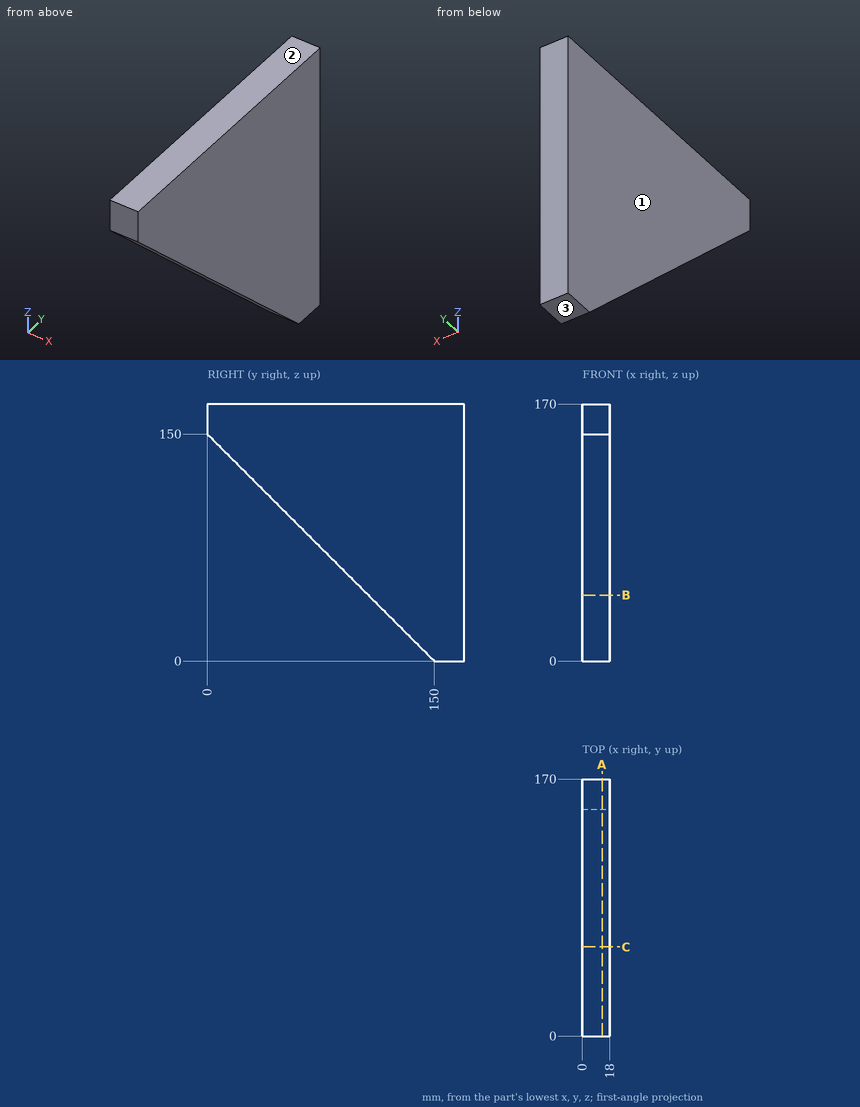
Geometry: see drawing. Coordinates: mm, zero at the bounding-box minimum. Coordinates: 2 decimals unless noted, no trailing zeros. Loops run counter-clockwise (first coordinate to the right, second up) from the corner with the lowest first, then second, coordinate; pieces in that order, holes last. Notation, with made-up numbers: (48.5, 10) -> (73.5, 10) arc R17 cw to (73.5, 32) -> close; hole circle Ø11 at (-3.5, 55). An arc over 180 degrees is marked (long way). Use a Markdown table: item, result.
1) Contact query for flat-ended pins moving along their axis: pin 1 (4 mm diameter, centred on x = 10.5, y = 113.5, fed in from -Z); pin 2 (2 mm diameter, centred on x = 2, z = 75, fed in from -Y). Output: stop coordinate, or through.
Results found:
| item | result |
|---|---|
| pin 1 | stops at z = 34.5 |
| pin 2 | stops at y = 74 |
2) Material intervals for line 1 along Z through (x, y) = (11.25, 123.5); line 2 along Y through (x, z) = (9.5, 37); line 3 along Z through (x, y) = (10.25, 16), sorted ascending. Write a range as from..to.
Results found:
| item | result |
|---|---|
| line 1 | z = 26.5..170 |
| line 2 | y = 113..170 |
| line 3 | z = 134..170 |
3) Pull-direction query (Z, two-part tool) for the marked faces 1, 2 and 3; classes: released by +Z, released by -Z, zero draft, split by the parting line, or undercut.
Results found:
| item | result |
|---|---|
| face 1 | zero draft |
| face 2 | released by +Z |
| face 3 | released by -Z |
4) Cut plane A-A (x = 13). Return the cut outline in (y, z).
Results found:
| item | result |
|---|---|
| outline | (0, 150) -> (150, 0) -> (170, 0) -> (170, 170) -> (0, 170) -> close |
5) Cut plane C-C (y = 59). Return the cut outline in (x, z).
Results found:
| item | result |
|---|---|
| outline | (0, 91) -> (18, 91) -> (18, 170) -> (0, 170) -> close |
6) Cut plane B-B (z = 43.5). Return the cut outline in (x, y).
Results found:
| item | result |
|---|---|
| outline | (0, 106.5) -> (18, 106.5) -> (18, 170) -> (0, 170) -> close |
